Check sheet for the modelled part. Datum: model origin and axes. Units: mm. Face numbers are marked on the shaded views. A direction names the side the tool comes from. Round coordinates to 2 decimals unless told otherwise and drop trailing zeros. Order: outer loops, then holes, each group sorted by start corner. A loop starts at its lowest first (then second) coordinate and runs counter-clockwise, first axis right, second up.
(1) Tool access check on the marked faces 1, 2, 3 and 4. Record the directions out of +Z, -Z, +X, -X, +Y, -Y that give a thin tool (end or side, any length) a straight path to the whole face; none if there is none.
(2) Mould release check, pull along X, two halves, no side actions. Record for the marked faces 5, 6, 7 and 8: released by +X, released by -X, zero draft, split by the parting line, or undercut.
(3) Sectioned sample at D-D, the plane y = 3.5. Enter the section's corners in (x, z), and give its area (3 significant figures).
(4) Sectioned sample at C-C, the plane z = 12.5. Enter the section's corners in (x, y) (3 decimals).
(5) Sectioned sample at B-B, the plane y = -5. Enter the section's corners in (x, z), and give its area (3 significant figures).
(6) Depth check by flat-ended pin: pin 1 (3.5 mm diameter, centred on x = 0, y = 12.975, fed in from +Z); pin 2 (4.5 mm diameter, centred on y = 12.86, z = 0, fed in from +X); pin 3 (2 mm diameter, centred on x = 12, z = -1.5, fed in from +Y); pin 4 (1.5 mm diameter, centred on x = 1, y = 6, fed in from +Z). Enter the tip coordinate at first touch or a pass-through.
(7) Thickness scan on probe 1 along Y at (x, z) = (16, 0); probe 2 along Y at (x, z) = (8, 0); probe 3 along X at (y, z) = (1, 0). Record the ranges inside material, lowest first.
(8) Sectioned sample at A-A, the plane z = 0. Enter the section's corners in (x, y), and give its area (3 significant figures).
```python
from build123d import *

# Parameters (mm, degrees)
SKETCH1_R              = 15
SKETCH1_R_2            = 4.5
BOSS_EXTRUDE1_DEPTH    = 9
SKETCH2_W              = 39.8
SKETCH2_H              = 30
BOSS_EXTRUDE2_DEPTH    = 7.95
M5_TAPPED_HOLE1_REACH  = 45.286
M5_TAPPED_HOLE1_BORE_R = 2.1
M5_TAPPED_HOLE2_REACH  = 45.286
M5_TAPPED_HOLE2_BORE_R = 2.1
SKETCH3_R              = 2.75
CUT_EXTRUDE1_DEPTH     = 40.790859579
SKETCH35_W             = 8
SKETCH35_H             = 4
SKETCH35_W_2           = 4
SKETCH35_H_2           = 8
CUT_EXTRUDE4_DEPTH     = 8
SKETCH40_R             = 2.75
CUT_EXTRUDE5_DEPTH     = 12


with BuildPart() as part:
    # Sketch1 → Boss-Extrude1 (new, symmetric)
    with BuildSketch(Plane(origin=(0, 0, 0), x_dir=(1, 0, 0), z_dir=(0, 1, 0))):
        with Locations(Location((0, 0, 0), (0, 0, 270))):
            Circle(SKETCH1_R)
        with Locations(Location((0, 0, 0), (0, 0, 270))):
            Circle(SKETCH1_R_2, mode=Mode.SUBTRACT)
    extrude(amount=BOSS_EXTRUDE1_DEPTH, both=True)

    # Sketch2 → Boss-Extrude2 (add)
    with BuildSketch(Plane(origin=(0, 9, 0), x_dir=(1, 0, 0), z_dir=(0, 1, 0))):
        Rectangle(SKETCH2_W, SKETCH2_H)
    extrude(amount=BOSS_EXTRUDE2_DEPTH)

    # M5 Tapped Hole1 bore → M5 Tapped Hole1 (cut, up to next)
    with BuildSketch(Plane(origin=(10.606601718, 0, -10.606601718), x_dir=(-0.7071067811865476, 0, -0.7071067811865476), z_dir=(0.7071067811865476, 0, -0.7071067811865476)), mode=Mode.PRIVATE) as m5_tapped_hole1_sk1:
        with Locations((0, -4)):
            Circle(M5_TAPPED_HOLE1_BORE_R)
    m5_tapped_hole1_tool1 = extrude(m5_tapped_hole1_sk1.sketch, amount=-M5_TAPPED_HOLE1_REACH, mode=Mode.PRIVATE) & part.part
    add(m5_tapped_hole1_tool1.solids().sort_by_distance((10.606602, -4, -10.606602))[0], mode=Mode.SUBTRACT)

    # M5 Tapped Hole2 bore → M5 Tapped Hole2 (cut, up to next)
    with BuildSketch(Plane(origin=(-10.606601718, 0, -10.606601718), x_dir=(-0.7071067811865476, 0, 0.7071067811865476), z_dir=(-0.7071067811865476, 0, -0.7071067811865476)), mode=Mode.PRIVATE) as m5_tapped_hole2_sk1:
        with Locations((0, -4)):
            Circle(M5_TAPPED_HOLE2_BORE_R)
    m5_tapped_hole2_tool1 = extrude(m5_tapped_hole2_sk1.sketch, amount=-M5_TAPPED_HOLE2_REACH, mode=Mode.PRIVATE) & part.part
    add(m5_tapped_hole2_tool1.solids().sort_by_distance((-10.606602, -4, -10.606602))[0], mode=Mode.SUBTRACT)

    # Sketch3 → Cut-Extrude1 (cut, through all)
    with BuildSketch(Plane(origin=(0, 0, -15), x_dir=(-1, 0, 0), z_dir=(0, 0, -1))):
        with Locations((0, 12.975)):
            Circle(SKETCH3_R)
    extrude(amount=-CUT_EXTRUDE1_DEPTH, mode=Mode.SUBTRACT)

    # Sketch35 → Cut-Extrude4 (cut)
    with BuildSketch(Plane(origin=(0, 16.95, 0), x_dir=(1, 0, 0), z_dir=(0, 1, 0))):
        Rectangle(SKETCH35_W, SKETCH35_H)
        with Locations((11.9, 0)):
            Rectangle(SKETCH35_W_2, SKETCH35_H_2)
    extrude(amount=-CUT_EXTRUDE4_DEPTH, mode=Mode.SUBTRACT)

    # Sketch40 → Cut-Extrude5 (cut)
    with BuildSketch(Plane(origin=(19.9, 0, 0), x_dir=(0, 0, -1), z_dir=(1, 0, 0))):
        with Locations((0, 12.8625)):
            Circle(SKETCH40_R)
    extrude(amount=-CUT_EXTRUDE5_DEPTH, mode=Mode.SUBTRACT)


solid = part.part
```
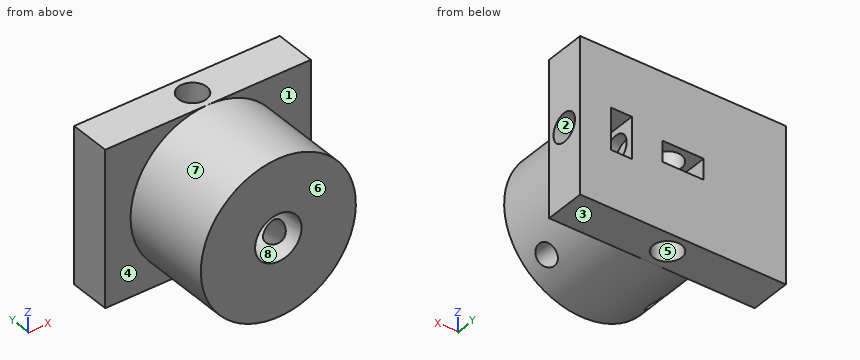
Derived:
1. face 1: +X, -Y
1. face 2: +X
1. face 3: -Z, +X, -X, +Y, -Y
1. face 4: -X, -Y
2. face 5: undercut
2. face 6: zero draft
2. face 7: split by the parting line
2. face 8: undercut
3. outline: circle Ø30 at (0, 0); hole circle Ø9 at (0, 0)
3. area: 643 mm2
4. outline: (-19.9, 9) - (-8.292, 9) - (-8.292, -9) - (8.292, -9) - (8.292, 9) - (19.9, 9) - (19.9, 16.95) - (-19.9, 16.95) - close; hole circle Ø5.5 at (0, 12.975)
5. outline: (-11.83, -9.22) - (-4.21, -1.6) arc R4.5 cw (long way) to (4.21, -1.6) - (11.83, -9.22) arc R15 ccw (long way) to start; (-9.22, -11.83) arc R15 ccw to (9.22, -11.83) - (1.6, -4.21) arc R4.5 cw to (-1.6, -4.21) - close
5. area: 565 mm2
6. pin 1: passes through
6. pin 2: stops at x = 7.9
6. pin 3: stops at y = 8.95
6. pin 4: stops at z = 15
7. probe 1: y = 9 to 10.11, 15.61 to 16.95
7. probe 2: y = -9 to 10.11, 15.61 to 16.95
7. probe 3: x = -15 to -4.5, 4.5 to 15
8. outline: (-19.9, 9) - (-15, 9) - (-15, -9) - (-4.5, -9) - (-4.5, 9) - (-4, 9) - (-4, 16.95) - (-19.9, 16.95) - close; (4, 9) - (4.5, 9) - (4.5, -9) - (15, -9) - (15, 9) - (19.9, 9) - (19.9, 10.11) - (13.9, 10.11) - (13.9, 8.95) - (9.9, 8.95) - (9.9, 10.11) - (7.9, 10.11) - (7.9, 15.61) - (9.9, 15.61) - (9.9, 16.95) - (4, 16.95) - close; (13.9, 15.61) - (19.9, 15.61) - (19.9, 16.95) - (13.9, 16.95) - close
8. area: 555 mm2
